Source: CAD feature listing. Evaluate the final solid. Frame: model axes, mm. Face numbers are marked on the shaded views. Coordinates: 2 decimals unless noted, no trailing zeros. Order: outer loops, then holes, each group sorted by start corner. A loop starts at its lowest first (then second) coordinate and runs counter-clockwise, first axis right, second up. Notation, with made-up numbers: (46.25, 68) -> (58.25, 68) arc R27 ccw to (58.25, 88) -> close; hole circle Ø7 at (45.5, 55). An arc over 180 degrees is marked (long way). Write each question's results on one line, items separated by ' | '. Start each with the question number.
from build123d import *

# Parameters (mm, degrees)
F0_R     = 15
F0_R_2   = 10
F1_DEPTH = 4
F0_R_3   = 7.5
F2_DEPTH = 10
F3_R     = 1


with BuildPart() as f1:
    # F0 (on Top) → F1 (new body)
    with BuildSketch(Plane.XY):
        Circle(F0_R)
        Circle(F0_R_2, mode=Mode.SUBTRACT)
    extrude(amount=F1_DEPTH)

    # F0 (on Top) → F2 (join)
    with BuildSketch(Plane.XY):
        Circle(F0_R_2)
        Circle(F0_R_3, mode=Mode.SUBTRACT)
    extrude(amount=F2_DEPTH)

    # F3
    f3_edges = [f1.edges().sort_by_distance(p)[0] for p in [
        (-7.5, 0, 10),
        (-10, 0, 10),
    ]]
    fillet(f3_edges, radius=F3_R)


solid = f1.part
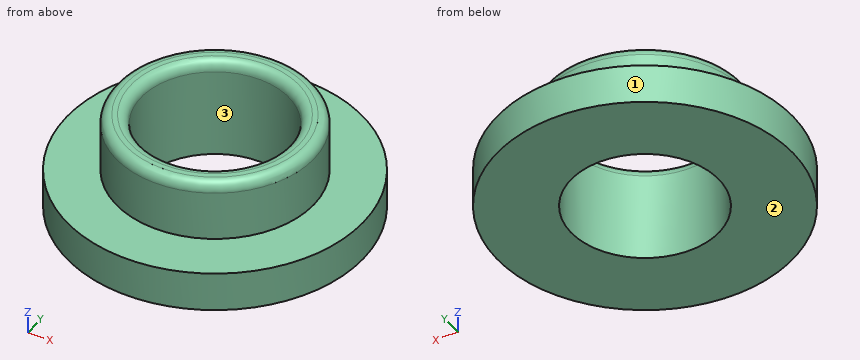
(1) First-contact query: P1, Ø1, axis at x = -8.5, z = 8, coming from the +Y side; P2, Ø1.5, axis at x = 8.5, z = 4, coming from the -Y side; P3, Ø5, axis at x = 12, z = 1, coming from the +Y side. Flat tips, straight axial feed; report the tip coordinate or a pass-through.
(2) Line query: L1, parallel to Y at x = 0, z = 2.75; L2, parallel to Z at x = 12, y = -5; L3, parallel to Y at x = 0, z = 6.25. Output: solid intervals per line, ascending.
(3) Section A-A on y = 0. Return the cut outline in (x, z).
(4) Draft query along Y for the marked faces 1, 2 and 3. Return one class per face: released by +Y, released by -Y, zero draft, split by the parting line, or undercut.
(5) Section D-D on y = 13. Return the cut outline in (x, z).
(6) Section C-C on z = 8.5. Return the cut outline in (x, y), then the cut area to 3 significant figures.
Results list:
1) P1: stops at y = 6 | P2: stops at y = -12.84 | P3: stops at y = 11.61
2) L1: y = -15 to -7.5, 7.5 to 15 | L2: z = 0 to 4 | L3: y = -10 to -7.5, 7.5 to 10
3) outline: (-15, 0) -> (-7.5, 0) -> (-7.5, 9) arc R1 ccw to (-8.5, 10) -> (-9, 10) arc R1 ccw to (-10, 9) -> (-10, 4) -> (-15, 4) -> close; (7.5, 0) -> (15, 0) -> (15, 4) -> (10, 4) -> (10, 9) arc R1 ccw to (9, 10) -> (8.5, 10) arc R1 ccw to (7.5, 9) -> close
4) face 1: split by the parting line | face 2: zero draft | face 3: undercut
5) outline: (-7.48, 0) -> (7.48, 0) -> (7.48, 4) -> (-7.48, 4) -> close
6) outline: circle Ø20 at (0, 0); hole circle Ø15 at (0, 0) | area: 137 mm²
